from build123d import *

# Parameters (mm, degrees)
SKETCH5_R                            = 1.8
BOSS_EXTRUDE2_DEPTH                  = 3
SKETCH6_W                            = 50
SKETCH6_H                            = 55
BOSS_EXTRUDE3_DEPTH                  = 3
M3_3_6MM_D                           = 3.6
MIRROR1_AT_THE_SECOND_PLANE_COPY_1_D = 3.6
BOSS_EXTRUDE4_DEPTH                  = 5
CHAMFER1_SIZE                        = 5


with BuildPart() as part:
    # Sketch5 → Boss-Extrude2 (new body)
    with BuildSketch(Plane.XY):
        with BuildLine():
            Line((0, 0), (0, 35))
            ThreePointArc((0, 35), (25, 60), (50, 35))
            Line((50, 35), (50, 0))
            Line((50, 0), (0, 0))
        make_face()
        with Locations((16.5, 35)):
            Circle(SKETCH5_R, mode=Mode.SUBTRACT)
        with Locations((33.5, 35)):
            Circle(SKETCH5_R, mode=Mode.SUBTRACT)
        with BuildLine():
            Line((28.65, 42.5), (28.65, 27.5))
            ThreePointArc((28.65, 27.5), (25, 23.85), (21.35, 27.5))
            Line((21.35, 27.5), (21.35, 42.5))
            ThreePointArc((21.35, 42.5), (25, 46.15), (28.65, 42.5))
        make_face(mode=Mode.SUBTRACT)
    extrude(amount=BOSS_EXTRUDE2_DEPTH)

    # Sketch6 → Boss-Extrude3 (add)
    with BuildSketch(Plane.XZ):
        with Locations((25, 27.5)):
            Rectangle(SKETCH6_W, SKETCH6_H)
    extrude(amount=-BOSS_EXTRUDE3_DEPTH)

    # M3, 3.6mm (through all)
    with Locations(Plane.XZ):
        with Locations((10, 42.5)):
            m3_3_6mm = Hole(M3_3_6MM_D / 2)

    # Mirror1: M3, 3.6mm across plane
    add(m3_3_6mm.mirror(Plane.ZY.offset(-25)), mode=Mode.SUBTRACT)

    # Mirror1 at the second plane: M3, 3.6mm across plane
    add(m3_3_6mm.mirror(Plane.XY.offset(27.5)), mode=Mode.SUBTRACT)

    # Mirror1 at the second plane copy 1 (through all)
    with Locations(Plane(origin=(50, 0, 55), x_dir=(-1, 0, 0), z_dir=(0, -1, 0))):
        with Locations((10, 42.5)):
            Hole(MIRROR1_AT_THE_SECOND_PLANE_COPY_1_D / 2)

    # Sketch10 → Boss-Extrude4 (add)
    with BuildSketch(Plane(origin=(50, 0, 0), x_dir=(0, 0, -1), z_dir=(1, 0, 0))):
        Polygon((-3, 35), (-55, 3), (-45.459789048, 3), (-3, 29.129100953), align=None)
    boss_extrude4 = extrude(amount=-BOSS_EXTRUDE4_DEPTH)

    # Mirror2: Boss-Extrude4 across plane
    add(boss_extrude4.mirror(Plane.ZY.offset(-25)))

    # Chamfer1
    chamfer1_edges = [part.edges().sort_by_distance(p)[0] for p in [
        (25, 3, 3),
    ]]
    chamfer(chamfer1_edges, length=CHAMFER1_SIZE)


solid = part.part
Part model, mm, in its own coordinate system. A direction names the side the tool comes from. Give positions to 0.01 mm unless a question says otherwise; leave off trailing zeros. Loops run counter-clockwise (first coordinate to the right, second up) from the corner with the lowest first, then second, coordinate; pieces in that order, holes last.
(1) Band-saw the part on B-B (z = 22.5). Write the cut outline in (x, y).
Return value:
outline: (0, 0) - (50, 0) - (50, 3) - (0, 3) - close; (0, 17.13) - (5, 17.13) - (5, 23) - (0, 23) - close; (45, 17.13) - (50, 17.13) - (50, 23) - (45, 23) - close
(2) Drill centre lines: line 1 along Z through (x, y) = (10, 1.5); line 2 along X through (y, z) = (2, 42); line 3 along X through (y, z) = (17.5, 24). Where is each one in solid material? Low to high.
Return value:
line 1: z = 0 to 10.7, 14.3 to 40.7, 44.3 to 55
line 2: x = 0 to 8.27, 11.73 to 38.27, 41.73 to 50
line 3: x = 0 to 5, 45 to 50
(3) 3-axis set-ups, long thin cutter, end or side, ignore diameter. For faces 4 (the flat face through (21.35, 35, 1)), 5 (the flat face through (25, 1, 55)), 6 (the flat face through (45, 17, 27)), 7 (the flat face through (47.5, 15.9, 24.5)): which of +Z, -Z, +X, -X, +Y, -Y reach the whole face in a straight line?
Return value:
face 4: +Z, -Z
face 5: +Z, +X, -X, +Y, -Y
face 6: +Z, +Y
face 7: +X, -X
(4) Band-saw the part on D-D (y = 25). Write the cut outline in (x, z).
Return value:
outline: (0, 0) - (22.34, 0) - (22.34, 3) - (0, 3) - close; (0, 9.71) - (5, 9.71) - (5, 19.25) - (0, 19.25) - close; (27.66, 0) - (50, 0) - (50, 3) - (27.66, 3) - close; (45, 9.71) - (50, 9.71) - (50, 19.25) - (45, 19.25) - close
(5) Pull direction Z, two halves, no side cores. Call faces 1 (the flat face through (28.65, 35, 1)), 2 (the flat face through (20, 30, 0)), 3 (the cylindrical face through (40.831, 1.521, 14.097)): pulls with the +Z half, pulls with the -Z half, needs draft (parallel to the pull), parting line crosses it, or undercut.
Return value:
face 1: needs draft
face 2: pulls with the -Z half
face 3: undercut
(6) Band-saw the part on C-C (x = 10). Write the cut outline in (y, z).
Return value:
outline: (0, 0) - (55, 0) - (55, 3) - (8, 3) - (3, 8) - (3, 10.7) - (0, 10.7) - close; (0, 14.3) - (3, 14.3) - (3, 40.7) - (0, 40.7) - close; (0, 44.3) - (3, 44.3) - (3, 55) - (0, 55) - close
(7) Band-saw the part on A-A (x = 25). Write the cut outline in (y, z), and give its area (3 significant figures).
Return value:
outline: (0, 0) - (23.85, 0) - (23.85, 3) - (8, 3) - (3, 8) - (3, 55) - (0, 55) - close; (46.15, 0) - (60, 0) - (60, 3) - (46.15, 3) - close
area: 282 mm2
(8) Pin check, flat tips, straight feed: pin 1 (3 mm diameter, centred on x = 40, z = 42.5, fed in from -Y); pin 2 (4.5 mm diameter, centred on x = 10, z = 42.5, fed in from +Y); pin 3 (0.9 mm diameter, centred on y = 36.5, z = 1.5, fed in from +X); pin 4 (8 mm diameter, centred on x = 21, y = 13, fed in from +Z). Stop position of each tip, or through.
Return value:
pin 1: passes through
pin 2: stops at y = 3
pin 3: stops at x = 49.98
pin 4: stops at z = 3
